from build123d import *

# Parameters (mm, degrees)
SKETCH1_W                = 25.2
SKETCH1_H                = 26
SKETCH1_R                = 1
SKETCH1_R_2              = 0.5
BOSS_EXTRUDE1_DEPTH      = 1.4
SKETCH2_W                = 24.6
SKETCH2_H                = 16.4
BOSS_EXTRUDE2_DEPTH      = 0.9
SKETCH3_W                = 10.16
SKETCH3_H                = 2.54
BOSS_EXTRUDE3_DEPTH      = 1
BOSS_EXTRUDE4_DEPTH      = 8.6
BOSS_EXTRUDE4_DEPTH_BACK = 2.7
SKETCH4_W                = 0.7
SKETCH4_H                = 0.7
CHAMFER1_SIZE            = 0.3
SKETCH5_W                = 21.744
SKETCH5_H                = 10.864
BOSS_EXTRUDE5_DEPTH      = 0.01


with BuildPart() as part:
    # Sketch1 → Boss-Extrude1 (new body)
    with BuildSketch(Plane(origin=(0, 0, 0), x_dir=(1, 0, 0), z_dir=(0, 1, 0))):
        Rectangle(SKETCH1_W, SKETCH1_H)
        with Locations(Location((-9.9, 11, 0), (0, 0, 270))):
            Circle(SKETCH1_R, mode=Mode.SUBTRACT)
        with Locations(Location((10.6, 11, 0), (0, 0, 270))):
            Circle(SKETCH1_R, mode=Mode.SUBTRACT)
        with Locations(Location((-9.9, -10.6, 0), (0, 0, 270))):
            Circle(SKETCH1_R, mode=Mode.SUBTRACT)
        with Locations(Location((10.6, -10.6, 0), (0, 0, 270))):
            Circle(SKETCH1_R, mode=Mode.SUBTRACT)
        with Locations(Location((-3.81, 11.75, 0), (0, 0, 270))):
            Circle(SKETCH1_R_2, mode=Mode.SUBTRACT)
        with Locations(Location((-1.27, 11.75, 0), (0, 0, 270))):
            Circle(SKETCH1_R_2, mode=Mode.SUBTRACT)
        with Locations(Location((1.27, 11.75, 0), (0, 0, 270))):
            Circle(SKETCH1_R_2, mode=Mode.SUBTRACT)
        with Locations(Location((3.81, 11.75, 0), (0, 0, 270))):
            Circle(SKETCH1_R_2, mode=Mode.SUBTRACT)
    extrude(amount=BOSS_EXTRUDE1_DEPTH)

    # Sketch2 → Boss-Extrude2 (add)
    with BuildSketch(Plane(origin=(0, 1.4, 0), x_dir=(1, 0, 0), z_dir=(0, 1, 0))):
        with Locations((0, 0.3)):
            Rectangle(SKETCH2_W, SKETCH2_H)
    extrude(amount=BOSS_EXTRUDE2_DEPTH)

    # Sketch3 → Boss-Extrude3 (add)
    with BuildSketch(Plane.XZ):
        with Locations((0, -11.75)):
            Rectangle(SKETCH3_W, SKETCH3_H)
    extrude(amount=BOSS_EXTRUDE3_DEPTH)

    # Sketch4 → Boss-Extrude4 (add, two sides: drawn at the far end of the back side and taken through both)
    with BuildSketch(Plane.XZ.offset(-BOSS_EXTRUDE4_DEPTH_BACK)):
        with Locations((-3.81, -11.75)):
            Rectangle(SKETCH4_W, SKETCH4_H)
        with Locations((-1.27, -11.75)):
            Rectangle(SKETCH4_W, SKETCH4_H)
        with Locations((1.27, -11.75)):
            Rectangle(SKETCH4_W, SKETCH4_H)
        with Locations((3.81, -11.75)):
            Rectangle(SKETCH4_W, SKETCH4_H)
    extrude(amount=BOSS_EXTRUDE4_DEPTH + BOSS_EXTRUDE4_DEPTH_BACK)

    # Chamfer1
    chamfer1_edges = [part.edges().sort_by_distance(p)[0] for p in [
        (-0.92, 2.7, -11.75),
        (-1.27, 2.7, -12.1),
        (-1.62, 2.7, -11.75),
        (-1.27, 2.7, -11.4),
        (-0.92, -8.6, -11.75),
        (-1.27, -8.6, -11.4),
        (-1.62, -8.6, -11.75),
        (-1.27, -8.6, -12.1),
        (1.62, 2.7, -11.75),
        (1.27, 2.7, -12.1),
        (0.92, 2.7, -11.75),
        (1.27, 2.7, -11.4),
        (1.62, -8.6, -11.75),
        (1.27, -8.6, -11.4),
        (0.92, -8.6, -11.75),
        (1.27, -8.6, -12.1),
        (4.16, 2.7, -11.75),
        (3.81, 2.7, -12.1),
        (3.46, 2.7, -11.75),
        (3.81, 2.7, -11.4),
        (4.16, -8.6, -11.75),
        (3.81, -8.6, -11.4),
        (3.46, -8.6, -11.75),
        (3.81, -8.6, -12.1),
        (-3.46, 2.7, -11.75),
        (-3.81, 2.7, -12.1),
        (-4.16, 2.7, -11.75),
        (-3.81, 2.7, -11.4),
        (-3.46, -8.6, -11.75),
        (-3.81, -8.6, -11.4),
        (-4.16, -8.6, -11.75),
        (-3.81, -8.6, -12.1),
    ]]
    chamfer(chamfer1_edges, length=CHAMFER1_SIZE)

    # Sketch5 → Boss-Extrude5 (add)
    with BuildSketch(Plane.XZ):
        with Locations((0, -1.198)):
            Rectangle(SKETCH5_W, SKETCH5_H)
    extrude(amount=BOSS_EXTRUDE5_DEPTH)


solid = part.part
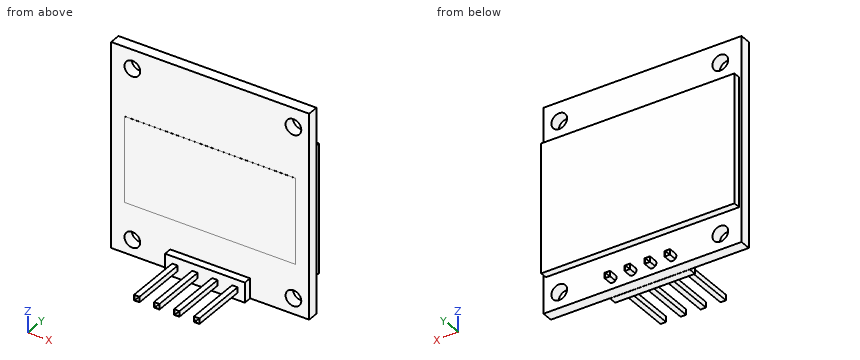
For this review, take the finished solid that the model builds, in its own axes (mm). Coordinates: 2 decimals unless noted, no trailing zeros. Order: outer loops, then holes, each group sorted by start corner. A loop starts at its lowest first (then second) coordinate and runs counter-clockwise, first axis right, second up. Notation, with made-up numbers: (6.5, -22) -> (44.5, -22) arc R18 cw to (44.5, -5) -> close; hole circle Ø2 at (-15.75, -34). An arc over 180 degrees is marked (long way). Return JSON: item names as keys, results as strings.
1. We need section B-B on z = 10.6. Write out the cut boundary in (x, y).
Answer block:
{"outline": "(-12.6, 0) -> (-10.9, 0) -> (-10.9, 1.4) -> (-12.6, 1.4) -> close; (-8.9, 0) -> (9.6, 0) -> (9.6, 1.4) -> (-8.9, 1.4) -> close; (11.6, 0) -> (12.6, 0) -> (12.6, 1.4) -> (11.6, 1.4) -> close"}
2. We need section D-D on z = -7. Write out the cut boundary in (x, y).
Answer block:
{"outline": "(-12.6, 0) -> (12.6, 0) -> (12.6, 1.4) -> (12.3, 1.4) -> (12.3, 2.3) -> (-12.3, 2.3) -> (-12.3, 1.4) -> (-12.6, 1.4) -> close"}
3. For line 1 (X direction, y = 0.65, z = -11); line 2 (X direction, y = -2.5, z = -12); line 3 (Y direction, x = 5.25, z = -6.5), list the stretches that pass through material, from the lowest coordinate up. Write a range as from..to.
Answer block:
{"line 1": "-12.6..-10.9, -8.9..9.6, 11.6..12.6", "line 2": "-4.16..-3.46, -1.62..-0.92, 0.92..1.62, 3.46..4.16", "line 3": "-0.01..2.3"}
4. We need section A-A on x = -9.9. State how many separate pieces and enclosed holes the cut face has, and give its area (3 significant figures).
Answer block:
{"separate pieces": "3", "enclosed holes": "0", "area": "45.7 mm²"}
5. For pin 1 Ø1.5 at (x, z) = (-8, 8) entering from -Y; pin 2 Ø0.8 at (y, z) = (-0.5, -12) entering from +X; pin 3 Ø4 at (x, z) = (-9.5, 1.5) entering from +Y, all flat-tipped, find the tip position at first contact; note any pin that passes through.
Answer block:
{"pin 1": "y = 0", "pin 2": "x = 5.08", "pin 3": "y = 2.3"}
